```python
from build123d import *

# Parameters (mm, degrees)
ESQUISSE1_R        = 30
ESQUISSE1_R_2      = 13
BOSS_EXTRU_1_DEPTH = 4.75
BOSS_EXTRU_2_START = -4.75
BOSS_EXTRU_2_DEPTH = 4.75
BOSS_EXTRU_3_DEPTH = 4.75


with BuildPart() as part:
    # Esquisse1 → Boss.-Extru.1 (new body)
    with BuildSketch(Plane(origin=(0, 0, 0), x_dir=(1, 0, 0), z_dir=(0, 1, 0))):
        with Locations(Location((0, 0, 0), (0, 0, 270))):
            Circle(ESQUISSE1_R)
        with Locations(Location((0, 0, 0), (0, 0, 270))):
            Circle(ESQUISSE1_R_2, mode=Mode.SUBTRACT)
        with BuildLine():
            ThreePointArc((-2.834733548, 23.018019494), (0.874151367, 16.41695293), (6.655356686, 11.527415922))
            ThreePointArc((6.655356686, 11.527415922), (10.753432897, 12.625492134), (9.655356686, 16.723568345))
            ThreePointArc((9.655356686, 16.723568345), (5.500346376, 20.237727687), (2.834733548, 24.981980506))
            ThreePointArc((2.834733548, 24.981980506), (-0.981980506, 26.834733548), (-2.834733548, 23.018019494))
        make_face(mode=Mode.SUBTRACT)
        with BuildLine():
            ThreePointArc((23.052396529, 10.036038988), (22.748570703, 14.267786838), (18.516822853, 13.963961012))
            ThreePointArc((18.516822853, 13.963961012), (14.654573974, 7.451439174), (13.310713372, 0))
            ThreePointArc((13.310713372, 0), (16.310713372, -3), (19.310713372, 0))
            ThreePointArc((19.310713372, 0), (20.27655948, 5.355424153), (23.052396529, 10.036038988))
        make_face(mode=Mode.SUBTRACT)
        with BuildLine():
            ThreePointArc((20.217662981, -14.945941518), (23.730551209, -12.56694671), (21.3515564, -9.054058482))
            ThreePointArc((21.3515564, -9.054058482), (13.780422607, -8.965513756), (6.655356686, -11.527415922))
            ThreePointArc((6.655356686, -11.527415922), (5.557280474, -15.625492134), (9.655356686, -16.723568345))
            ThreePointArc((9.655356686, -16.723568345), (14.776213104, -14.882303535), (20.217662981, -14.945941518))
        make_face(mode=Mode.SUBTRACT)
        with BuildLine():
            ThreePointArc((-2.834733548, -24.981980506), (0.981980506, -26.834733548), (2.834733548, -23.018019494))
            ThreePointArc((2.834733548, -23.018019494), (-0.874151367, -16.41695293), (-6.655356686, -11.527415922))
            ThreePointArc((-6.655356686, -11.527415922), (-10.753432897, -12.625492134), (-9.655356686, -16.723568345))
            ThreePointArc((-9.655356686, -16.723568345), (-5.500346376, -20.237727687), (-2.834733548, -24.981980506))
        make_face(mode=Mode.SUBTRACT)
        with BuildLine():
            ThreePointArc((-23.052396529, -10.036038988), (-22.748570703, -14.267786838), (-18.516822853, -13.963961012))
            ThreePointArc((-18.516822853, -13.963961012), (-14.654573974, -7.451439174), (-13.310713372, 0))
            ThreePointArc((-13.310713372, 0), (-16.310713372, 3), (-19.310713372, 0))
            ThreePointArc((-19.310713372, 0), (-20.27655948, -5.355424153), (-23.052396529, -10.036038988))
        make_face(mode=Mode.SUBTRACT)
        with BuildLine():
            ThreePointArc((-20.217662981, 14.945941518), (-23.730551209, 12.56694671), (-21.3515564, 9.054058482))
            ThreePointArc((-21.3515564, 9.054058482), (-13.780422607, 8.965513756), (-6.655356686, 11.527415922))
            ThreePointArc((-6.655356686, 11.527415922), (-5.557280474, 15.625492134), (-9.655356686, 16.723568345))
            ThreePointArc((-9.655356686, 16.723568345), (-14.776213104, 14.882303535), (-20.217662981, 14.945941518))
        make_face(mode=Mode.SUBTRACT)
    extrude(amount=BOSS_EXTRU_1_DEPTH)

    # Esquisse2 → Boss.-Extru.2 (add)
    with BuildSketch(Plane(origin=(0, 4.75, 0), x_dir=(1, 0, 0), z_dir=(0, 1, 0)).offset(BOSS_EXTRU_2_START)):
        with BuildLine():
            Line((19.448716719, 22.841791041), (20.183832184, 22.215874605))
            ThreePointArc((20.183832184, 22.215874605), (25.759295996, 19.87106259), (31.666737758, 21.169550915))
            Line((31.666737758, 21.169550915), (44.657118814, 28.669550915))
            ThreePointArc((44.657118814, 28.669550915), (48.072182324, 27.754487405), (47.157118814, 24.339423896))
            Line((47.157118814, 24.339423896), (34.166737758, 16.839423896))
            ThreePointArc((34.166737758, 16.839423896), (29.989946446, 12.152392884), (29.430081471, 5.899361893))
            Line((29.430081471, 5.899361893), (29.20996886, 6.839423896))
            ThreePointArc((29.20996886, 6.839423896), (25.611244779, 15.622552316), (19.448716719, 22.841791041))
        make_face()
    extrude(amount=BOSS_EXTRU_2_DEPTH)

    # Esquisse3 → Boss.-Extru.3 (add)
    with BuildSketch(Plane(origin=(0, 4.75, 0), x_dir=(1, 0, 0), z_dir=(0, 1, 0))):
        Polygon((34.599750459, 17.089423896), (36.909151536, 17.089423896), (36.331801267, 18.089423896), align=None)
        Polygon((40.661928286, 20.589423896), (42.393979093, 21.589423896), (41.239278555, 19.589423896), align=None)
    extrude(amount=-BOSS_EXTRU_3_DEPTH)


solid = part.part
```
CAD build for the part. Positions are in the model's coordinates, mm. A direction names the side the tool comes from. Round coordinates to 2 decimals unless told otherwise and drop trailing zeros. Write each loop counter-clockwise with the first axis right and the second up, starting at its lowest first coordinate (ties: lowest second). Pieces come first, ordered by that corner, then holes. Notation, with made-up numbers: (-39, 14) -> (18, 14) arc R18 cw to (18, 48) -> close; hole circle Ø4 at (-25.75, 52). An arc over 180 degrees is marked (long way). Answer in a Markdown table with one row per item. Add a question column.
Item 1: Saw through at C-C, the plane y = 3.55. Count the separate pieces of the cut face and the enclosed holes in it, then the cut area to 3 significant figures.
Item 2: Drill centre lines: line 1 (Z direction, x = 6, y = 2.7); line 2 (X direction, y = 1.85, z = -12); line 3 (X direction, y = 3.95, z = 5). Where is each one in solid material? Low to high. Write a range as from..to.
Item 3: Saw through at B-B, the plane z = 7. Write the cut outline in (x, y), then the cut area to 3 significant figures.
Item 4: Drop a flat-ended pin along its axis: pin 1 Ø1.5 at (x, y) = (-5, 1.5) entering from +Z. Give the stop position or say it passes through.
Item 5: Saw through at A-A, the plane x = 0. Write the cut outline in (y, z).
Item 6: Mould opens along X. For faces 1 (the face through (44.809, 2.342, -22.984)), 2 (the face through (12, 0, -7)), 3 (the face through (10.72, 2.34, -12.57)) say: pulls with the +X half, pulls with the -X half, needs draft (parallel to the pull), parting line crosses it, or undercut.
Item 7: Which spindle directions (+Z, -Z, +X, -X, +Y, -Y) get a long thin tool onto all of the face, cutting with end or side? Do faces 4 (the face through (38.071, 2.342, -24.867)), 5 (the face through (14.69, 2.34, -7.55)), 6 (the face through (12, 4.75, -7)). Say none if no direction does.
Item 8: Saw through at D-D, the plane x = 38.5. Write the cut outline in (y, z).
Findings below:
| question | item | result |
|---|---|---|
| 1 | separate pieces | 1 |
| 1 | enclosed holes | 7 |
| 1 | area | 1,810 mm^2 |
| 2 | line 1 | z = -29.39..-19.66, -11.92..-11.53, 11.53..12.04, 16.21..29.39 |
| 2 | line 2 | x = -27.5..-23.78, -6.04..-5, 5..5.88, 10.27..17.01, 23.78..29.93 |
| 2 | line 3 | x = -29.58..-20.15, -13.91..-12, 12..29.58 |
| 3 | outline | (-29.17, 0) -> (-21, 0) -> (-21, 4.75) -> (-29.17, 4.75) -> close; (-14.49, 0) -> (-10.95, 0) -> (-10.95, 4.75) -> (-14.49, 4.75) -> close; (10.95, 0) -> (29.17, 0) -> (29.17, 4.75) -> (10.95, 4.75) -> close |
| 3 | area | 142 mm^2 |
| 4 | pin 1 | stops at z = 29.7 |
| 5 | outline | (0, -30) -> (4.75, -30) -> (4.75, -27) -> (0, -27) -> close; (0, -17.55) -> (4.75, -17.55) -> (4.75, -13) -> (0, -13) -> close; (0, 13) -> (4.75, 13) -> (4.75, 17.55) -> (0, 17.55) -> close; (0, 27) -> (4.75, 27) -> (4.75, 30) -> (0, 30) -> close |
| 6 | face 1 | pulls with the +X half |
| 6 | face 2 | needs draft |
| 6 | face 3 | undercut |
| 7 | face 4 | -Z, +Y, -Y |
| 7 | face 5 | +Y, -Y |
| 7 | face 6 | +Z, -Z, +X, -X, +Y |
| 8 | outline | (0, -25.11) -> (4.75, -25.11) -> (4.75, -19.34) -> (0, -19.34) -> close |
